Work out the finished part from the listing and answer in its coordinate system (mm). A direction names the side the tool comes from. Round coordinates to 2 decimals unless told otherwise and drop trailing zeros. Write each loop counter-clockwise with the first axis right and the second up, starting at its lowest first coordinate (ties: lowest second). Pieces come first, ordered by that corner, then holes. Notation, with made-up numbers: (-6.75, -36.5) -> (40.25, -36.5) arc R14 cw to (40.25, -23.5) -> close; hole circle Ø9 at (21.5, -37.75). An arc over 180 degrees is marked (long way). One line per item, written item: value.
```python
from build123d import *

# Parameters (mm, degrees)
F1_W      = 126.9999492
F1_H      = 127.0000508
F2_DEPTH  = 10.16
F3_W      = 114.2999492
F3_H      = 114.3000508
F4_DEPTH  = 10.161
F5_W      = 10.4391968
F5_H      = 51.0824988
F5_W_2    = 15.240254
F5_H_2    = 6.35
F5_W_3    = 19.531076
F6_DEPTH  = 10.161
F7_W      = 6.3186603262
F7_H      = 12.6597918
F8_DEPTH  = 10.16
F10_D     = 2.3749
F11_R     = 1.18745
F12_DEPTH = 2.794
F15_W     = 12.7
F15_H     = 26.589482
F16_DEPTH = 10.16
F15_H_2   = 10.1803962
F18_D     = 3.4544
F18_DEPTH = 6.35
F18_TIP   = 1.0378064612
F9_W      = 6.35
F9_H      = 18.117566
F9_W_2    = 30.48
F9_H_2    = 6.35
F9_W_3    = 8.1742328233
F9_H_3    = 3.990848
F19_DEPTH = 3.81
F20_W     = 45.6544562851
F20_H     = 1.059942
F21_DEPTH = 10.161
F22_W     = 53.3058220283
F22_H     = 3.769614
F22_W_2   = 15.240254
F22_H_2   = 2.629916
F23_DEPTH = 3.81
F24_W     = 6.379972
F24_H     = 12.6597918
F25_DEPTH = 2.54


# Not quite as in the source:
# - a feature names something its author has since deleted; it is built from what else it names


with BuildPart() as f2:
    # F1 (on Top) → F2 (new body)
    with BuildSketch(Plane.XY):
        with Locations((0.1398778, 0)):
            Rectangle(F1_W, F1_H)
    extrude(amount=-F2_DEPTH)

    # F3 (on face) → F4 (cut, through all)
    with BuildSketch(Plane(origin=(0, 0, -10.16), x_dir=(1, 0, 0), z_dir=(0, 0, -1))):
        with Locations((0.1398778, 0)):
            Rectangle(F3_W, F3_H)
    extrude(amount=-F4_DEPTH, mode=Mode.SUBTRACT)

    # F5 (on face) → F6 (cut, through all)
    with BuildSketch(Plane(origin=(0, 0, -10.16), x_dir=(1, 0, 0), z_dir=(0, 0, -1))):
        with Locations((-58.420254, 37.958776)):
            Rectangle(F5_W, F5_H)
        with Locations((-43.7761126, -60.3250254)):
            Rectangle(F5_W_2, F5_H_2)
        with Locations((53.8743144, 60.3250254)):
            Rectangle(F5_W_3, F5_H_2)
    extrude(amount=-F6_DEPTH, mode=Mode.SUBTRACT)


with BuildPart() as f8:
    # F7 (on face) → F8 (new body)
    with BuildSketch(Plane(origin=(0, 0, -10.16), x_dir=(1, 0, 0), z_dir=(0, 0, -1))):
        Polygon((-37.8689406421, 34.3098374), (-37.8689406421, 46.9696292), (-31.5502803159, 46.9696292), (-31.5502803159, 57.1500254), (-44.2886084, 57.1500254), (-44.2886084, 34.3098374), align=None)
        with Locations((-34.709610479, 40.6397333)):
            Rectangle(F7_W, F7_H)
        Polygon((57.2898524, 46.9696292), (-31.5502803159, 46.9696292), (-31.5502803159, 34.3098374), (31.9114424, 34.3098374), (44.5713104, 34.3098374), (57.2898524, 34.3098374), align=None)
        Polygon((44.5713104, 34.3098374), (31.9114424, 34.3098374), (31.9114424, -23.2499154), (31.9114424, -29.2427535486), (31.9114424, -30.5605434), (31.9114424, -41.8902134), (31.9114424, -57.1500254), (44.5713104, -57.1500254), align=None)
        Polygon((31.9114424, -29.2427535486), (31.9114424, -23.2499154), (-57.0100968, -23.2499154), (-57.0100968, -30.5605434), (31.9114424, -30.5605434), align=None)
    extrude(amount=-F8_DEPTH)

    # F10 (through all)
    with Locations(Plane.XY):
        with Locations((38.2398524, 35.5602794), (38.2398524, -40.639746), (-37.9601476, -40.639746)):
            Hole(F10_D / 2)

    # F11 (on face) → F12 (cut)
    with BuildSketch(Plane(origin=(0, 0, -10.16), x_dir=(1, 0, 0), z_dir=(0, 0, -1))):
        Polygon((-34.2943619493, 40.693121057), (-36.17347893, 43.8410970268), (-39.8392645806, 43.7877219698), (-41.6259332507, 40.586370943), (-39.74681627, 37.4383949732), (-36.0810306194, 37.4917700302), align=None)
        with Locations((-37.9601476, 40.639746)):
            Circle(F11_R, mode=Mode.SUBTRACT)
        Polygon((34.5740667493, 40.586370943), (36.45318373, 37.4383949732), (40.1189693806, 37.4917700302), (41.9056380507, 40.693121057), (40.02652107, 43.8410970268), (36.3607354194, 43.7877219698), align=None)
        Polygon((36.3607354194, -32.4123034302), (34.5740667493, -35.613654457), (36.45318373, -38.7616304268), (40.1189693806, -38.7082553698), (41.9056380507, -35.506904343), (40.02652107, -32.3589283732), align=None)
    extrude(amount=-F12_DEPTH, mode=Mode.SUBTRACT)

    # F14: union F2
    add(f2.part)


with BuildPart() as f16:
    # F15 (on face) → F16 (new body, through all)
    with BuildSketch(Plane.XY):
        with Locations((2.6457252283, 43.8552844)):
            Rectangle(F15_W, F15_H)
    extrude(amount=-F16_DEPTH)


with BuildPart() as f16b:
    # F15 (on face) → F16, piece 2 (new body, through all)
    with BuildSketch(Plane.XY):
        with Locations((37.7587764, -52.0598273)):
            Rectangle(F15_W, F15_H_2)
    extrude(amount=-F16_DEPTH)


with BuildPart() as f16_1:
    add(f16.part)

    # F17: union F16b, F8
    add(f16b.part)
    add(f8.part)

    # F18
    with Locations(Plane(origin=(0, 0, -10.16), x_dir=(1, 0, 0), z_dir=(0, 0, -1))):
        with Locations((0.1805810421, 40.6397333), (-4.5459396, 60.3250254), (-60.1850968, -25.6824734), (38.2398524, -60.3250254), (60.4648524, -38.1000254), (60.4648524, 31.7500254)):
            Hole(F18_D / 2, depth=F18_DEPTH)
            with Locations((0, 0, -(F18_DEPTH + F18_TIP / 2))):  # 118° drill point
                Cone(0, F18_D / 2, F18_TIP, mode=Mode.SUBTRACT)

    # F9 (on face) → F19 (cut)
    with BuildSketch(Plane.XY):
        with Locations((-60.1850968, 47.2840304)):
            Rectangle(F9_W, F9_H)
        with Locations((-16.3704016, 60.3250254)):
            Rectangle(F9_W_2, F9_H_2)
        with Locations((47.8253068116, 59.1454494)):
            Rectangle(F9_W_3, F9_H_3)
    extrude(amount=-F19_DEPTH, mode=Mode.SUBTRACT)

    # F20 (on face) → F21 (cut, through all)
    with BuildSketch(Plane.XY):
        with Locations((-4.2932037426, 23.7798864)):
            Rectangle(F20_W, F20_H)
    extrude(amount=-F21_DEPTH, mode=Mode.SUBTRACT)

    # F22 (on face) → F23 (join)
    with BuildSketch(Plane.XY):
        with Locations((-30.3571857859, 32.4453504)):
            Rectangle(F22_W, F22_H)
        with Locations((-43.7761126, 62.1850674)):
            Rectangle(F22_W_2, F22_H_2)
    extrude(amount=-F23_DEPTH)

    # F24 (on face) → F25 (cut)
    with BuildSketch(Plane.XY):
        with Locations((-17.7036476, -40.6397333)):
            Rectangle(F24_W, F24_H)
    extrude(amount=-F25_DEPTH, mode=Mode.SUBTRACT)


solid = f16_1.part
```
(1) Find section A-A on y = -23. Give the vertices of the cut face in (x, z).
Reported:
outline: (31.91, -10.16) -> (44.57, -10.16) -> (44.57, 0) -> (31.91, 0) -> close; (57.29, -10.16) -> (63.64, -10.16) -> (63.64, 0) -> (57.29, 0) -> close
(2) For a pull along X with two mould halves and no side action, classify faces 1 (the face through (-17, 60, -3.81)), 2 (the face through (-60, 56.343, -2)) as pulls with the +X half, pulls with the -X half, needs draft (parallel to the pull), parting line crosses it, or undercut.
Reported:
face 1: undercut
face 2: needs draft
(3) Find section B-B on x = 25. Give the vertices of the cut face in (y, z).
Reported:
outline: (-63.5, -10.16) -> (-57.15, -10.16) -> (-57.15, 0) -> (-63.5, 0) -> close; (-46.97, -10.16) -> (-34.31, -10.16) -> (-34.31, 0) -> (-46.97, 0) -> close; (23.25, -10.16) -> (30.56, -10.16) -> (30.56, 0) -> (23.25, 0) -> close; (57.15, -10.16) -> (63.5, -10.16) -> (63.5, 0) -> (57.15, 0) -> close
(4) A tool of negligible diameter and unlimited length cuts with its end or side. For faces 3 (the face through (-36.156, 60, -6)), 4 (the face through (-60, 47, -3.81)), 5 (the face through (13, 29, 0)), 6 (the face through (48, 59, -3.81)), 7 (the face through (44.109, -55, -5)), from which of +Z, -Z, +X, -X, +Y, -Y can it reach the whole face along a straight path? Write none if from no direction.
Reported:
face 3: -Z
face 4: +Z, -X
face 5: +Z, +X, -X, +Y, -Y
face 6: +Z
face 7: +Z, -Z, -Y
(5) Find section C-C on y = -53.5. Give the vertices of the cut face in (x, z), plus the area to 3 significant figures.
Reported:
outline: (-44.29, -10.16) -> (-31.55, -10.16) -> (-31.55, 0) -> (-44.29, 0) -> close; (31.41, -10.16) -> (44.11, -10.16) -> (44.11, 0) -> (31.41, 0) -> close; (57.29, -10.16) -> (63.64, -10.16) -> (63.64, 0) -> (57.29, 0) -> close
area: 323 mm2
(6) Consider probe 1 along Y at (x, z) = (-18, -4.25); probe 2 along Y at (x, z) = (20.5, -4.5); probe 3 along X at (y, z) = (-3, -1.5). Determine where each line is inside the solid, lowest interval first.
Reported:
probe 1: y = -63.5 to -57.15, -46.97 to -34.31, 24.31 to 30.56, 57.15 to 63.5
probe 2: y = -63.5 to -57.15, -46.97 to -34.31, 23.25 to 30.56, 57.15 to 63.5
probe 3: x = -63.36 to -57.01, 31.91 to 44.57, 57.29 to 63.64
(7) Flat-ended cylindrical pins translate along their axes: pin 1 Ø5.5 at (x, y) = (60.46, -31.75) entering from +Z; pin 2 Ø6 at (y, z) = (-36, -2) entering from -X; pin 3 Ø3 at (x, z) = (-61.5, -2) entering from -Y; pin 4 Ø1.1 at (x, y) = (-40.5, 31.5) entering from -Z. Find the tip coordinate at first contact, or state that the pin passes through.
Reported:
pin 1: stops at z = 0
pin 2: stops at x = -44.29
pin 3: stops at y = -12.42
pin 4: stops at z = -3.81
(8) Find section D-D on y = 48.5. Give the vertices of the cut face in (x, z), plus the area to 3 significant figures.
Reported:
outline: (-63.36, -10.16) -> (-57.01, -10.16) -> (-57.01, -3.81) -> (-63.36, -3.81) -> close; (-3.7, -10.16) -> (9, -10.16) -> (9, 0) -> (-3.7, 0) -> close; (31.91, -10.16) -> (44.57, -10.16) -> (44.57, 0) -> (31.91, 0) -> close; (57.29, -10.16) -> (63.64, -10.16) -> (63.64, 0) -> (57.29, 0) -> close
area: 362 mm2
